The listing builds one solid part. Answer for the finished solid, in the listing's coordinates (mm). A direction names the side the tool comes from. Coordinates: 2 decimals unless noted, no trailing zeros. Order: outer loops, then holes, each group sorted by start corner. A loop starts at its lowest first (then second) coordinate and runs counter-clockwise, first axis right, second up. Notation, with made-up numbers: (-21.5, -6) -> (-11.5, -6) arc R21 cw to (-11.5, 27) -> close; hole circle Ø6 at (34.25, 46). An arc over 180 degrees is marked (long way). Write each question's results on one line, items separated by ' | '. Start each with the question number.
(1) Straight lines are drawn through the part: L1, parallel to X at y = 50.8, z = 2 (3 decimals); L2, parallel to Y at x = 17.5, z = 26; L3, parallel to Z at x = 21.5, y = -31 (3 decimals). For each, find the intervals that lie inside material, in ascending order.
(2) The part is cut by section C-C, the plane y = -37.5. Give the vertices of the cut face in (x, z) (3 decimals), then the cut area to 3 significant figures.
(3) A tool of negligible diameter and unlimited length cuts with its end or side. For faces 5 (the face through (46, -25.4, 42)), 6 (the face through (45.9, -0.4, 38.2)), 7 (the face through (46, 25.4, 42)), 8 (the face through (22.225, -17, 18)), 9 (the face through (80, -6, 38.1)), from which of +Z, -Z, +X, -X, +Y, -Y can it reach the whole face along a straight path? Write none if from no direction.
(4) The part is cut by section B-B, the plane z = 3. Give the vertices of the cut face in (x, y) (3 decimals), then the cut area to 3 significant figures.
(5) Determine the mould class of faces 1 (the face through (-26.12, -48.55, 5.95)), 2 (the face through (28.988, -47.652, -1.984)), 3 (the face through (22.225, 17, 18)), 4 (the face through (-39.464, -61.59, -0.133)) for opening direction Y: +Y half, -Y half, draft (parallel to the pull), parting line (faces both ways), or undercut.
(6) The part is cut by section A-A, the plane y = -50.8. Give the vertices of the cut face in (x, z) (3 decimals).
(7) Given pin 1 (4 mm diameter, centred on x = 28.575, y = -50.8, fed in from +Z); pin 2 (1.5 mm diameter, centred on x = -15, y = -18, fed in from +Z) (3 decimals); pin 3 (7.5 mm diameter, centred on x = -28.575, y = 50.8, fed in from -Z) (3 decimals); pin 4 (8.5 mm diameter, centred on y = -21, z = 19, fed in from -X) (3 decimals), each flat-ended and moving along its own axis, determine where each tip first touches the part or whether it passes through.
```python
from build123d import *

# Parameters (mm, degrees)
F1_DEPTH        = 63.5
F0_W            = 25.4
F0_H            = 19.05
F2_DEPTH        = 25.4
F3_DEPTH        = 7.9375
F5_R            = 6.35
F6_R            = 7.9375
F7_DEPTH        = 38.1
F8_SIZE         = 2.54
F10_D           = 6.35
F10_CSINK_D     = 12.8778
F10_CSINK_ANGLE = 82


with BuildPart() as f1:
    # F0 (on Front) → F1 (new body, symmetric)
    with BuildSketch(Plane.XZ):
        Polygon((-41.275, -9.525), (41.275, -9.525), (41.275, 9.525), (22.225, 9.525), (-41.275, 9.525), align=None)
    extrude(amount=F1_DEPTH, both=True)

    # F0 (on Front) → F2 (join, symmetric)
    with BuildSketch(Plane.XZ):
        with Locations((73.025, 52.4002)):
            Rectangle(F0_W, F0_H)
        with BuildLine():
            Line((22.225, 9.525), (41.275, 9.525))
            Line((41.275, 9.525), (41.275, 27.0021876939))
            ThreePointArc((41.275, 27.0021876939), (46.0138493613, 38.3159745909), (57.401207742, 42.8752))
            Line((57.401207742, 42.8752), (60.325, 42.8752))
            Line((60.325, 42.8752), (60.325, 61.9252))
            Line((60.325, 61.9252), (57.5226076573, 61.9252))
            add(Edge.make_bspline(
                [(56.7269681039, 61.9246255958), (56.9914748423, 61.9259537401), (57.2566863526, 61.9261483453), (57.5226076573, 61.9252)],
                knots=[111.1760466233, 111.1760466233, 111.1760466233, 111.1760466233, 111.8335738446, 111.8335738446, 111.8335738446, 111.8335738446], degree=3))
            ThreePointArc((56.7269681039, 61.9246255958), (32.3051814862, 51.5478719991), (22.225, 27.0021876939))
            Line((22.225, 27.0021876939), (22.225, 9.525))
        make_face()
    extrude(amount=F2_DEPTH, both=True)

    # F0 (on Front) → F3 (join, symmetric)
    with BuildSketch(Plane.XZ):
        with BuildLine():
            add(Edge.make_bspline(
                [(-41.275, 9.525), (-12.5711712421, 29.0690447456), (12.0036281031, 61.7000602517), (56.7269681039, 61.9246255958)],
                knots=[0, 0, 0, 0, 111.1760466233, 111.1760466233, 111.1760466233, 111.1760466233], degree=3))
            Line((-41.275, 9.525), (22.225, 9.525))
            Line((22.225, 9.525), (22.225, 27.0021876939))
            ThreePointArc((22.225, 27.0021876939), (32.3051814862, 51.5478719991), (56.7269681039, 61.9246255958))
        make_face()
    extrude(amount=F3_DEPTH, both=True)

    # F0 (on Front) → F4 (revolve)
    with BuildSketch(Plane.XZ):
        Polygon((85.725, 61.9252), (85.725, 42.8752), (85.725, 38.1), (111.125, 38.1), (111.125, 66.675), (85.725, 66.675), align=None)
    revolve(axis=Axis((85.725, 0, 52.3875), (0, 0, -1)))

    # F5
    f5_edges = [f1.edges().sort_by_distance(p)[0] for p in [
        (41.275, -63.5, 0),
        (-41.275, -63.5, 0),
        (-41.275, 63.5, 0),
        (41.275, 63.5, 0),
    ]]
    fillet(f5_edges, radius=F5_R)

    # F6 (on face) → F7 (cut, symmetric)
    with BuildSketch(Plane.XY.offset(66.675)):
        with Locations((85.725, 0)):
            Circle(F6_R)
    extrude(amount=F7_DEPTH, both=True, mode=Mode.SUBTRACT)

    # F8
    f8_edges = [f1.edges().sort_by_distance(p)[0] for p in [
        (77.7875, 0, 66.675),
    ]]
    chamfer(f8_edges, length=F8_SIZE)

    # F10 (through all)
    with Locations(Plane.XY.offset(9.525)):
        with Locations((-28.575, 50.8), (28.575, 50.8), (28.575, -50.8), (-28.575, -50.8)):
            CounterSinkHole(F10_D / 2, F10_CSINK_D / 2, counter_sink_angle=F10_CSINK_ANGLE)


solid = f1.part
```
Established:
1) L1: x = -41.275 to -31.75, -25.4 to 25.4, 31.75 to 41.275 | L2: y = -7.94 to 7.94 | L3: z = -9.525 to 9.525
2) outline: (-41.275, -9.525) -> (41.275, -9.525) -> (41.275, 9.525) -> (-41.275, 9.525) -> close | area: 1,570 mm^2
3) face 5: +Z, +X, -X, -Y | face 6: -Z, +Y, -Y | face 7: +Z, +X, -X, +Y | face 8: +Z, -X, -Y | face 9: -Z, +X, +Y, -Y
4) outline: (-41.275, -57.15) arc R6.35 ccw to (-34.925, -63.5) -> (34.925, -63.5) arc R6.35 ccw to (41.275, -57.15) -> (41.275, 57.15) arc R6.35 ccw to (34.925, 63.5) -> (-34.925, 63.5) arc R6.35 ccw to (-41.275, 57.15) -> close; hole circle Ø6.35 at (-28.575, -50.8); hole circle Ø6.35 at (-28.575, 50.8); hole circle Ø6.35 at (28.575, -50.8); hole circle Ø6.35 at (28.575, 50.8) | area: 10,300 mm^2
5) face 1: undercut | face 2: undercut | face 3: draft | face 4: -Y half
6) outline: (-41.275, -9.525) -> (-31.75, -9.525) -> (-31.75, 5.77) -> (-35.014, 9.525) -> (-41.275, 9.525) -> close; (-25.4, -9.525) -> (25.4, -9.525) -> (25.4, 5.77) -> (22.136, 9.525) -> (-22.136, 9.525) -> (-25.4, 5.77) -> close; (31.75, -9.525) -> (41.275, -9.525) -> (41.275, 9.525) -> (35.014, 9.525) -> (31.75, 5.77) -> close
7) pin 1: passes through | pin 2: stops at z = 9.525 | pin 3: stops at z = -9.525 | pin 4: stops at x = 22.225
